Work out the finished part from the listing and answer in its coordinate system (mm). Give positions to 0.01 mm unless a question says otherwise; leave off trailing zeros. Order: outer loops, then holes, each group sorted by start corner. A loop starts at its lowest first (then second) coordinate and runs counter-clockwise, first axis right, second up. Notation, with made-up numbers: M 73.5,0 L 79.5,0 A5 ccw 79.5,5 Z; hole C 42.5,80.5 d7. An arc over 180 degrees is marked long. One line per item, written item: value.
from build123d import *

# Parameters (mm, degrees)
SKETCH1_R           = 1.6
SKETCH1_R_2         = 0.89
SKETCH1_2_R         = 1.6
SKETCH1_2_R_2       = 0.89
BOSS_EXTRUDE1_DEPTH = 6
SKETCH5_R           = 1.6
SKETCH5_R_2         = 0.89
BOSS_EXTRUDE2_DEPTH = 20


with BuildPart() as part:
    # Sweep1: sweep along a path in Sketch2
    with BuildLine(Plane(origin=(0, 0, 0), x_dir=(0, 0, -1), z_dir=(1, 0, 0))) as sweep1_path:
        ThreePointArc((0, 0), (-4.930222368, 2.030804149), (-6.99978301, 6.944883598))
    # Sketch1 → Sweep1 (sweep)
    with BuildSketch(Plane.XY):
        Circle(SKETCH1_R)
        Circle(SKETCH1_R_2, mode=Mode.SUBTRACT)
    sweep(path=sweep1_path.line)

    # Sketch1_2 → Boss-Extrude1 (add)
    with BuildSketch(Plane.XY):
        Circle(SKETCH1_2_R)
        Circle(SKETCH1_2_R_2, mode=Mode.SUBTRACT)
    extrude(amount=-BOSS_EXTRUDE1_DEPTH)

    # Sketch5 → Boss-Extrude2 (add)
    with BuildSketch(Plane(origin=(0, 6.999566026, 0.055114693), x_dir=(1, 0, 0), z_dir=(0, 0.999969001, 0.007873772))):
        with Locations((0, -6.944883598)):
            Circle(SKETCH5_R)
        with Locations((0, -6.944883598)):
            Circle(SKETCH5_R_2, mode=Mode.SUBTRACT)
    extrude(amount=BOSS_EXTRUDE2_DEPTH)


solid = part.part
(1) Find the intervals of material crossed by probe 1 along Y at (x, z) = (0, -2.75); probe 2 along Z at (x, y) = (0, 24.5); probe 3 along Y at (x, z) = (-0.3, -5.5), in increasing order. Write a range as from..to.
Findings:
probe 1: y = -1.6..-0.89, 0.89..1.6
probe 2: z = 5.54..6.25, 8.03..8.74
probe 3: y = -1.57..-0.84, 0.84..1.57
(2) Section A-A, the plane x = 0 is taken. Give the vertices of the cut face in (y, z).
Findings:
outline: M -1.6,-6 L -0.89,-6 L -0.89,0 A7.89 cw 6.94,7.89 L 26.94,8.05 L 26.93,8.76 L 6.93,8.6 A8.6 ccw -1.6,0 Z; M 0.89,-6 L 1.6,-6 L 1.6,0 A5.4 cw 6.96,5.4 L 26.96,5.56 L 26.95,6.27 L 6.95,6.11 A6.11 ccw 0.89,0 Z
(3) Determine the mould class of faces 1 (the flat face through (1, -1, -6)), 2 (the cylindrical face through (-0.116, 16.812, 6.195)), 3 (the cylindrical face through (-1.27, -0.97, -2.96)), 4 (the cylindrical face through (1.526, 16.808, 6.597)) for opening direction Z: pulls with the +Z half, pulls with the -Z half, needs draft (parallel to the pull), parting line crosses it, or undercut.
Findings:
face 1: pulls with the -Z half
face 2: undercut
face 3: needs draft
face 4: parting line crosses it
(4) Section B-B, the plane z = -2.75 is taken. Give the vertices of the cut face in (x, y).
Findings:
outline: C 0,0 d3.2; hole C 0,0 d1.78
(5) Given P1, Ø6, axis at y = 17.5, z = 3, coming from the -X side; P2, Ø1, axis at x = 1, z = 1.5, coming from the +Y side, each flat-ended and moving along its own axis, determine where each tip first touches the part or whether it passes through.
Findings:
P1: stops at x = -1.18
P2: stops at y = 1.79
